Input: part model. Units: mm. Frame: model coordinates. A direction names the side the tool comes from. Give positions to 0.01 mm unless a question says otherwise; leave off trailing zeros. Use a Markdown table: item, result.
from build123d import *

# Parameters (mm, degrees)
SKETCH1_R                    = 212.725
BOSS_EXTRUDE1_DEPTH          = 1.9939
SKETCH2_R                    = 19.05
SKETCH2_R_2                  = 7.62
SKETCH2_R_3                  = 34.925
CUT_EXTRUDE1_DEPTH           = 301.845187575
BOSS_EXTRUDE2_START          = -1.9939
BOSS_EXTRUDE2_DEPTH          = 1.9939
FILLET1_R                    = 25.4
F_1_4_CLEARANCE_HOLE2_D      = 6.7564
FILLET2_R                    = 6.35
BOSS_EXTRUDE3_START          = -1.9939
BOSS_EXTRUDE3_DEPTH          = 1.9939
F_3_8_0_405_DIAMETER_HOLE1_D = 9.525
CUT_EXTRUDE2_DEPTH           = 340.09265521
FILLET3_R                    = 22.86


with BuildPart() as part:
    # Sketch1 → Boss-Extrude1 (new body)
    with BuildSketch(Plane(origin=(0, 0, 0), x_dir=(1, 0, 0), z_dir=(0, 1, 0))):
        with Locations(Location((0, 0, 0), (0, 0, 270))):
            Circle(SKETCH1_R)
    extrude(amount=BOSS_EXTRUDE1_DEPTH)

    # Sketch2 → Cut-Extrude1 (cut, through all)
    with BuildSketch(Plane(origin=(0, 1.9939, 0), x_dir=(1, 0, 0), z_dir=(0, 1, 0))):
        with Locations(Location((0, 0, 0), (0, 0, 270))):
            Circle(SKETCH2_R)
        with Locations(Location((35.921024484, 0, 0), (0, 0, 270))):
            Circle(SKETCH2_R_2)
        with Locations(Location((0, 35.921024484, 0), (0, 0, 270))):
            Circle(SKETCH2_R_2)
        with BuildLine():
            ThreePointArc((-54.951572567, 5.210468059), (-44.180940607, 5.560163901), (-43.831244764, -5.210468059))
            Line((-43.831244764, -5.210468059), (-57.211826385, -19.489075291))
            ThreePointArc((-57.211826385, -19.489075291), (-67.982458345, -19.838771134), (-68.332154188, -9.068139174))
            Line((-68.332154188, -9.068139174), (-54.951572567, 5.210468059))
        make_face()
        with BuildLine():
            ThreePointArc((-9.068139174, -68.332154188), (-19.838771134, -67.982458345), (-19.489075291, -57.211826385))
            Line((-19.489075291, -57.211826385), (-5.210468059, -43.831244764))
            ThreePointArc((-5.210468059, -43.831244764), (5.560163901, -44.180940607), (5.210468059, -54.951572567))
            Line((5.210468059, -54.951572567), (-9.068139174, -68.332154188))
        make_face()
        with Locations((-63.221003092, -63.221003092)):
            Circle(SKETCH2_R_3)
        with BuildLine():
            ThreePointArc((-82.803000118, -92.139872667), (-87.916707425, -87.916707425), (-92.139872667, -82.803000118))
            ThreePointArc((-92.139872667, -82.803000118), (-95.549925128, -95.549925128), (-82.803000118, -92.139872667))
        make_face()
    extrude(amount=-CUT_EXTRUDE1_DEPTH, mode=Mode.SUBTRACT)

    # Sketch3 → Boss-Extrude2 (add)
    with BuildSketch(Plane(origin=(0, 1.9939, 0), x_dir=(1, 0, 0), z_dir=(0, 1, 0)).offset(BOSS_EXTRUDE2_START)):
        with BuildLine():
            Line((178.529712063, -115.667919216), (226.751467057, -163.88967421))
            ThreePointArc((226.751467057, -163.88967421), (226.751467057, -226.751467057), (163.88967421, -226.751467057))
            Line((163.88967421, -226.751467057), (115.667919216, -178.529712063))
            ThreePointArc((115.667919216, -178.529712063), (150.419290028, -150.419290028), (178.529712063, -115.667919216))
        make_face()
        with BuildLine():
            Line((-178.529712063, -115.667919216), (-226.751467057, -163.88967421))
            ThreePointArc((-226.751467057, -163.88967421), (-226.751467057, -226.751467057), (-163.88967421, -226.751467057))
            Line((-163.88967421, -226.751467057), (-115.667919216, -178.529712063))
            ThreePointArc((-115.667919216, -178.529712063), (-150.419290028, -150.419290028), (-178.529712063, -115.667919216))
        make_face()
        with BuildLine():
            Line((-115.667919216, 178.529712063), (-163.88967421, 226.751467057))
            ThreePointArc((-163.88967421, 226.751467057), (-226.751467057, 226.751467057), (-226.751467057, 163.88967421))
            Line((-226.751467057, 163.88967421), (-178.529712063, 115.667919216))
            ThreePointArc((-178.529712063, 115.667919216), (-150.419290028, 150.419290028), (-115.667919216, 178.529712063))
        make_face()
        with BuildLine():
            Line((178.529712063, 115.667919216), (226.751467057, 163.88967421))
            ThreePointArc((226.751467057, 163.88967421), (226.751467057, 226.751467057), (163.88967421, 226.751467057))
            Line((163.88967421, 226.751467057), (115.667919216, 178.529712063))
            ThreePointArc((115.667919216, 178.529712063), (150.419290028, 150.419290028), (178.529712063, 115.667919216))
        make_face()
    extrude(amount=BOSS_EXTRUDE2_DEPTH)

    # Fillet1
    fillet1_edges = [part.edges().sort_by_distance(p)[0] for p in [
        (115.667919216, 0.99695, 178.529712063),
        (178.529712063, 0.99695, 115.667919216),
        (-178.529712063, 0.99695, 115.667919216),
        (-115.667919216, 0.99695, 178.529712063),
        (-115.667919216, 0.99695, -178.529712063),
        (-178.529712063, 0.99695, -115.667919216),
        (178.529712063, 0.99695, -115.667919216),
        (115.667919216, 0.99695, -178.529712063),
    ]]
    fillet(fillet1_edges, radius=FILLET1_R)

    # 1/4 Clearance Hole2 (through all)
    with Locations(Plane(origin=(0, 1.9939, 0), x_dir=(1, 0, 0), z_dir=(0, 1, 0))):
        with Locations((-202.235367846, 156.974876996), (-224.686008149, 179.425517299), (-156.974876996, 202.235367846), (-179.425517299, 224.686008149), (202.235367846, -156.974876996), (224.686008149, -179.425517299), (156.974876996, -202.235367846), (179.425517299, -224.686008149), (224.686008149, 179.425517299), (202.235367846, 156.974876996), (179.425517299, 224.686008149), (156.974876996, 202.235367846), (-202.235367846, -156.974876996), (-224.686008149, -179.425517299), (-156.974876996, -202.235367846), (-179.425517299, -224.686008149), (49.391408666, -22.450640303), (-44.901280605, -107.763073453), (-107.763073453, -44.901280605), (-22.450640303, 49.391408666)):
            Hole(F_1_4_CLEARANCE_HOLE2_D / 2)

    # Fillet2
    fillet2_edges = [part.edges().sort_by_distance(p)[0] for p in [
        (-92.139872667, 0.99695, 82.803000118),
        (-82.803000118, 0.99695, 92.139872667),
    ]]
    fillet(fillet2_edges, radius=FILLET2_R)

    # Sketch12 → Boss-Extrude3 (add)
    with BuildSketch(Plane(origin=(0, 1.9939, 0), x_dir=(1, 0, 0), z_dir=(0, 1, 0)).offset(BOSS_EXTRUDE3_START)):
        with BuildLine():
            Line((-129.541916692, -192.40370954), (-149.863207153, -212.725))
            Line((-149.863207153, -212.725), (0, -212.725))
            ThreePointArc((0, -212.725), (-51.359035142, -206.432010924), (-99.679387975, -187.925371459))
            ThreePointArc((-99.679387975, -187.925371459), (-115.348395389, -185.245109949), (-129.541916692, -192.40370954))
        make_face()
        with BuildLine():
            ThreePointArc((99.679387975, -187.925371459), (51.359035142, -206.432010924), (0, -212.725))
            Line((0, -212.725), (149.863207153, -212.725))
            Line((149.863207153, -212.725), (129.541916692, -192.40370954))
            ThreePointArc((129.541916692, -192.40370954), (115.348395389, -185.245109949), (99.679387975, -187.925371459))
        make_face()
        with BuildLine():
            ThreePointArc((-187.925371459, -99.679387975), (-206.432010924, -51.359035142), (-212.725, 0))
            Line((-212.725, 0), (-212.725, -149.863207153))
            Line((-212.725, -149.863207153), (-192.40370954, -129.541916692))
            ThreePointArc((-192.40370954, -129.541916692), (-185.245109949, -115.348395389), (-187.925371459, -99.679387975))
        make_face()
        with BuildLine():
            Line((-192.40370954, 129.541916692), (-212.725, 149.863207153))
            Line((-212.725, 149.863207153), (-212.725, 0))
            ThreePointArc((-212.725, 0), (-206.432010924, 51.359035142), (-187.925371459, 99.679387976))
            ThreePointArc((-187.925371459, 99.679387976), (-185.245109949, 115.348395389), (-192.40370954, 129.541916692))
        make_face()
        with BuildLine():
            ThreePointArc((-99.679387975, 187.925371459), (-51.359035455, 206.432010847), (-6.44e-07, 212.725))
            Line((-6.44e-07, 212.725), (-149.863207153, 212.725))
            Line((-149.863207153, 212.725), (-129.541916692, 192.40370954))
            ThreePointArc((-129.541916692, 192.40370954), (-115.348395389, 185.245109949), (-99.679387975, 187.925371459))
        make_face()
        with BuildLine():
            Line((129.541916692, 192.40370954), (149.863207153, 212.725))
            Line((149.863207153, 212.725), (-6.44e-07, 212.725))
            ThreePointArc((-6.44e-07, 212.725), (51.35903483, 206.432011002), (99.679387976, 187.925371459))
            ThreePointArc((99.679387976, 187.925371459), (115.348395389, 185.245109949), (129.541916692, 192.40370954))
        make_face()
        with BuildLine():
            ThreePointArc((187.925371459, 99.679387975), (206.432011089, 51.35903448), (212.725, -1.365e-06))
            Line((212.725, -1.365e-06), (212.725, 149.863207153))
            Line((212.725, 149.863207153), (192.40370954, 129.541916692))
            ThreePointArc((192.40370954, 129.541916692), (185.245109949, 115.348395389), (187.925371459, 99.679387975))
        make_face()
        with BuildLine():
            Line((192.40370954, -129.541916692), (212.725, -149.863207153))
            Line((212.725, -149.863207153), (212.725, -1.365e-06))
            ThreePointArc((212.725, -1.365e-06), (206.43201076, -51.359035805), (187.925371459, -99.679387976))
            ThreePointArc((187.925371459, -99.679387976), (185.245109949, -115.348395389), (192.40370954, -129.541916692))
        make_face()
    extrude(amount=BOSS_EXTRUDE3_DEPTH)

    # 3/8 (0.405) Diameter Hole1 (through all)
    with Locations(Plane(origin=(0, 1.9939, 0), x_dir=(1, 0, 0), z_dir=(0, 1, 0))):
        with Locations((0, -142.875), (-142.875, 0), (142.875, 0), (0, 142.875)):
            Hole(F_3_8_0_405_DIAMETER_HOLE1_D / 2)

    # Sketch32 → Cut-Extrude2 (cut, through all)
    with BuildSketch(Plane(origin=(0, 1.9939, 0), x_dir=(1, 0, 0), z_dir=(0, 1, 0))):
        Polygon((-149.863207153, -212.725), (-145.100707153, -207.9625), (145.100707153, -207.9625), (149.863207153, -212.725), align=None)
        Polygon((-212.725, 149.863207153), (-207.9625, 145.100707153), (-207.9625, -145.100707153), (-212.725, -149.863207153), align=None)
        Polygon((149.863207153, 212.725), (145.100707153, 207.9625), (-145.100707153, 207.9625), (-149.863207153, 212.725), align=None)
        Polygon((212.725, -149.863207153), (207.9625, -145.100707153), (207.9625, 145.100707153), (212.725, 149.863207153), align=None)
    extrude(amount=-CUT_EXTRUDE2_DEPTH, mode=Mode.SUBTRACT)

    # Fillet3
    fillet3_edges = [part.edges().sort_by_distance(p)[0] for p in [
        (-145.100707153, 0.99695, 207.9625),
        (145.100707153, 0.99695, 207.9625),
        (-207.9625, 0.99695, -145.100707153),
        (-207.9625, 0.99695, 145.100707153),
        (145.100707153, 0.99695, -207.9625),
        (-145.100707153, 0.99695, -207.9625),
        (207.9625, 0.99695, 145.100707153),
        (207.9625, 0.99695, -145.100707153),
    ]]
    fillet(fillet3_edges, radius=FILLET3_R)


solid = part.part
1) First-contact query: pin 1 Ø1 at (y, z) = (1, 29.5) entering from -X; pin 2 Ø1 at (x, y) = (-145.5, 1.5) entering from -Z; pin 3 Ø1 at (y, z) = (1, -41.5) entering from +X. Flat tips, straight axial feed; report the tip coordinate or a pass-through.
Response values:
| item | result |
|---|---|
| pin 1 | stops at x = -207.96 |
| pin 2 | stops at z = -210.45 |
| pin 3 | stops at x = 207.96 |
2) Cut plane A-A on y = 0.9. State how many separate pieces and enclosed holes the cut face has, and give its area (3 significant figures).
Response values:
| item | result |
|---|---|
| separate pieces | 1 |
| enclosed holes | 30 |
| area | 180,000 mm² |
3) Reachability of faces 1 (the face through (-50.43, 1.01, 12.25)), 2 (the face through (-157.93, 0.98, 220.79)), 3 (the face through (220.62, 0.98, -157.76)), 4 (the face through (-220.62, 0.98, 157.76)) from +Z, -Z, +X, -X, +Y, -Y: full face, straight path, thin tool, end or side. Return the list, or none.
Response values:
| item | result |
|---|---|
| face 1 | +Y, -Y |
| face 2 | +Z, +Y, -Y |
| face 3 | +X, +Y, -Y |
| face 4 | -X, +Y, -Y |
4) Material intervals for line 1 (Z direction, x = -23, y = 1.8); line 2 (X direction, y = 1.5, z = -50); line 3 (X direction, y = 1, z = 60.5), sorted ascending. Write a range as from..to.
Response values:
| item | result |
|---|---|
| line 1 | z = -207.96..-52.72, -46.06..207.96 |
| line 2 | x = -207.96..-25.77, -19.13..207.96 |
| line 3 | x = -207.96..-98.04, -28.4..-21.55, -0.71..207.96 |
